Verification items for the finished model (mm, model axes). Face numbers are marked on the shaded views. A direction names the side the tool comes from. Give positions to 0.01 mm unless a question says otherwise; leave off trailing zeros. Write each loop counter-clockwise with the first axis right and the second up, starting at its lowest first coordinate (ties: lowest second). Pieces come first, ordered by that corner, then holes. Notation, with made-up numbers: (-14, -24) - (44, -24) arc R38 ccw to (44, 14) - close; hole circle Ø5 at (22.5, 31.5). An arc over 180 degrees is marked (long way). Answer as a JSON object with one key per item and string values. Group by question number.
Item 1: Sectioned sample at A-A, the plane x = -38. Record the boundary of the cut face in (y, z) (3 decimals), and give its area (3 significant figures).
Item 2: Draft check along Y on the marked faces 1, 2, 3 and 4. Enter one of: +Y half, -Y half, draft (parallel to the pull), parting line (faces both ways), or undercut.
Item 3: Scan lines: line 1 along Y through (x, z) = (-58, 29.5) (3 decimals); line 2 along Y through (x, z) = (-23, -48) (3 decimals); line 3 along X through (y, z) = (48.5, -33.5). Record each from-to range of solid material in increasing order. Write a range as [from, to].
Item 4: Sectioned sample at C-C, the plane x = -65.5. Record the boundary of the cut face in (y, z).
Item 5: Go/stop test with flat-tipped pins: pin 1 (1 mm diameter, centred on y = 69.5, z = 2, fed in from +X); pin 2 (16.5 mm diameter, centred on x = -52.39, z = 51.59, fed in from +Y); pin 3 (1.6 mm diameter, centred on y = 68.5, z = -47, fed in from +X) (3 decimals); pin 4 (7.5 mm diameter, centred on x = -28.58, z = 54.77, fed in from -Y). Record where each tip stops, or that it passes through.
Item 6: Tool access check on the marked faces 5 and 6. Record the directions out of +Z, -Z, +X, -X, +Y, -Y that give a thin tool (end or side, any length) a straight path to the whole face; none if there is none.
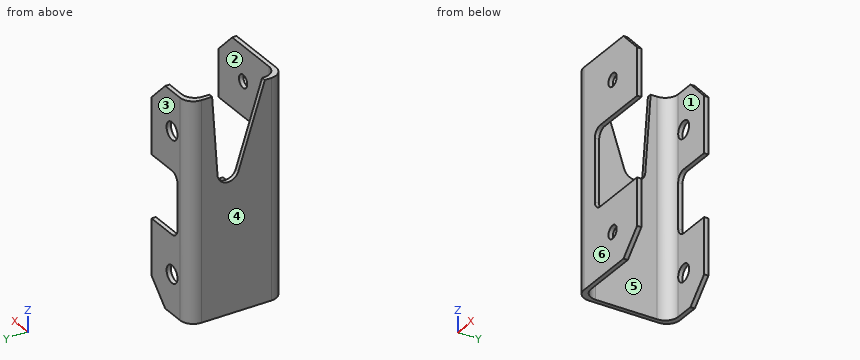
```python
from build123d import *

# Parameters (mm, degrees)
BOSS_EXTRUDE1_DEPTH = 80.16875
CUT_EXTRUDE2_DEPTH  = 4.175
CUT_EXTRUDE3_REACH  = 72.644
SKETCH3_R           = 6.35
CUT_EXTRUDE4_REACH  = 5.175
SKETCH4_R           = 4.7625


with BuildPart() as part:
    # Sketch1 → Boss-Extrude1 (new body, symmetric)
    with BuildSketch(Plane.XY):
        with BuildLine():
            Line((0, 0), (-61.9125, 0))
            ThreePointArc((-61.9125, 0), (-68.647692091, 2.789807909), (-71.4375, 9.525))
            Line((-71.4375, 9.525), (-71.4375, 61.11875))
            ThreePointArc((-71.4375, 61.11875), (-68.647692091, 67.853942091), (-61.9125, 70.64375))
            Line((-61.9125, 70.64375), (-28.575, 70.64375))
            Line((-28.575, 70.64375), (-28.575, 67.46875))
            Line((-28.575, 67.46875), (-58.7375, 67.46875))
            ThreePointArc((-58.7375, 67.46875), (-65.472692091, 64.678942091), (-68.2625, 57.94375))
            Line((-68.2625, 57.94375), (-68.2625, 12.7))
            ThreePointArc((-68.2625, 12.7), (-65.472692091, 5.964807909), (-58.7375, 3.175))
            Line((-58.7375, 3.175), (0, 3.175))
            Line((0, 3.175), (0, 0))
        make_face()
    extrude(amount=BOSS_EXTRUDE1_DEPTH, both=True)

    # Sketch2 → Cut-Extrude2 (cut, through all)
    with BuildSketch(Plane(origin=(-68.2625, 0, 0), x_dir=(0, 0, -1), z_dir=(1, 0, 0))):
        with BuildLine():
            Line((-22.471470052, 49.193610415), (-80.16875, 53.18125))
            Line((-80.16875, 53.18125), (-80.16875, 14.2875))
            Line((-80.16875, 14.2875), (-20.557643239, 33.728685684))
            ThreePointArc((-20.557643239, 33.728685684), (-15.141341042, 42.249850944), (-22.471470052, 49.193610415))
        make_face()
    extrude(amount=-CUT_EXTRUDE2_DEPTH, mode=Mode.SUBTRACT)

    # Sketch3 → Cut-Extrude3 (cut, up to next)
    with BuildSketch(Plane(origin=(0, 70.64375, 0), x_dir=(1, 0, 0), z_dir=(0, 1, 0)), mode=Mode.PRIVATE) as cut_extrude3_sk1:
        with Locations((-52.3875, 51.59375)):
            Circle(SKETCH3_R)
    cut_extrude3_tool1 = extrude(cut_extrude3_sk1.sketch, amount=-CUT_EXTRUDE3_REACH, mode=Mode.PRIVATE) & part.part
    add(cut_extrude3_tool1.solids().sort_by_distance((-52.3875, 70.64375, -51.59375))[0], mode=Mode.SUBTRACT)
    # Sketch3 → Cut-Extrude3 (cut, up to next)
    with BuildSketch(Plane(origin=(0, 70.64375, 0), x_dir=(1, 0, 0), z_dir=(0, 1, 0)), mode=Mode.PRIVATE) as cut_extrude3_sk2:
        with Locations((-52.3875, -51.59375)):
            Circle(SKETCH3_R)
    cut_extrude3_tool2 = extrude(cut_extrude3_sk2.sketch, amount=-CUT_EXTRUDE3_REACH, mode=Mode.PRIVATE) & part.part
    add(cut_extrude3_tool2.solids().sort_by_distance((-52.3875, 70.64375, 51.59375))[0], mode=Mode.SUBTRACT)
    # Sketch3 → Cut-Extrude3 (cut, up to next)
    with BuildSketch(Plane(origin=(0, 70.64375, 0), x_dir=(1, 0, 0), z_dir=(0, 1, 0)), mode=Mode.PRIVATE) as cut_extrude3_sk3:
        Polygon((-44.45, 80.16875), (-28.575, 64.29375), (-28.575, 80.16875), align=None)
    cut_extrude3_tool3 = extrude(cut_extrude3_sk3.sketch, amount=-CUT_EXTRUDE3_REACH, mode=Mode.PRIVATE) & part.part
    add(cut_extrude3_tool3.solids().sort_by_distance((-33.866667, 70.64375, -74.877083))[0], mode=Mode.SUBTRACT)
    # Sketch3 → Cut-Extrude3 (cut, up to next)
    with BuildSketch(Plane(origin=(0, 70.64375, 0), x_dir=(1, 0, 0), z_dir=(0, 1, 0)), mode=Mode.PRIVATE) as cut_extrude3_sk4:
        Polygon((-28.575, -80.16875), (-28.575, -64.29375), (-44.45, -80.16875), align=None)
    cut_extrude3_tool4 = extrude(cut_extrude3_sk4.sketch, amount=-CUT_EXTRUDE3_REACH, mode=Mode.PRIVATE) & part.part
    add(cut_extrude3_tool4.solids().sort_by_distance((-33.866667, 70.64375, 74.877083))[0], mode=Mode.SUBTRACT)
    # Sketch3 → Cut-Extrude3 (cut, up to next)
    with BuildSketch(Plane(origin=(0, 70.64375, 0), x_dir=(1, 0, 0), z_dir=(0, 1, 0)), mode=Mode.PRIVATE) as cut_extrude3_sk5:
        Polygon((-15.875, 80.16875), (0, 64.29375), (0, 80.16875), align=None)
    cut_extrude3_tool5 = extrude(cut_extrude3_sk5.sketch, amount=-CUT_EXTRUDE3_REACH, mode=Mode.PRIVATE) & part.part
    add(cut_extrude3_tool5.solids().sort_by_distance((-5.291667, 70.64375, -74.877083))[0], mode=Mode.SUBTRACT)
    # Sketch3 → Cut-Extrude3 (cut, up to next)
    with BuildSketch(Plane(origin=(0, 70.64375, 0), x_dir=(1, 0, 0), z_dir=(0, 1, 0)), mode=Mode.PRIVATE) as cut_extrude3_sk6:
        Polygon((-15.875, -80.16875), (0, -80.16875), (0, -64.29375), align=None)
    cut_extrude3_tool6 = extrude(cut_extrude3_sk6.sketch, amount=-CUT_EXTRUDE3_REACH, mode=Mode.PRIVATE) & part.part
    add(cut_extrude3_tool6.solids().sort_by_distance((-5.291667, 70.64375, 74.877083))[0], mode=Mode.SUBTRACT)
    # Sketch3 → Cut-Extrude3 (cut, up to next)
    with BuildSketch(Plane(origin=(0, 70.64375, 0), x_dir=(1, 0, 0), z_dir=(0, 1, 0)), mode=Mode.PRIVATE) as cut_extrude3_sk7:
        with BuildLine():
            Line((-28.575, 23.01875), (-28.575, -23.01875))
            Line((-28.575, -23.01875), (-52.3875, -23.01875))
            ThreePointArc((-52.3875, -23.01875), (-56.877628061, -21.158878061), (-58.7375, -16.66875))
            Line((-58.7375, -16.66875), (-58.7375, 16.66875))
            ThreePointArc((-58.7375, 16.66875), (-56.877628061, 21.158878061), (-52.3875, 23.01875))
            Line((-52.3875, 23.01875), (-28.575, 23.01875))
        make_face()
    cut_extrude3_tool7 = extrude(cut_extrude3_sk7.sketch, amount=-CUT_EXTRUDE3_REACH, mode=Mode.PRIVATE) & part.part
    add(cut_extrude3_tool7.solids().sort_by_distance((-43.483817, 70.64375, 0))[0], mode=Mode.SUBTRACT)

    # Sketch4 → Cut-Extrude4 (cut, up to next)
    with BuildSketch(Plane(origin=(0, 3.175, 0), x_dir=(1, 0, 0), z_dir=(0, 1, 0)), mode=Mode.PRIVATE) as cut_extrude4_sk1:
        with Locations((-28.575, 54.76875)):
            Circle(SKETCH4_R)
    cut_extrude4_tool1 = extrude(cut_extrude4_sk1.sketch, amount=-CUT_EXTRUDE4_REACH, mode=Mode.PRIVATE) & part.part
    add(cut_extrude4_tool1.solids().sort_by_distance((-28.575, 3.175, -54.76875))[0], mode=Mode.SUBTRACT)
    # Sketch4 → Cut-Extrude4 (cut, up to next)
    with BuildSketch(Plane(origin=(0, 3.175, 0), x_dir=(1, 0, 0), z_dir=(0, 1, 0)), mode=Mode.PRIVATE) as cut_extrude4_sk2:
        with Locations((-28.575, -54.76875)):
            Circle(SKETCH4_R)
    cut_extrude4_tool2 = extrude(cut_extrude4_sk2.sketch, amount=-CUT_EXTRUDE4_REACH, mode=Mode.PRIVATE) & part.part
    add(cut_extrude4_tool2.solids().sort_by_distance((-28.575, 3.175, 54.76875))[0], mode=Mode.SUBTRACT)
    # Sketch4 → Cut-Extrude4 (cut, up to next)
    with BuildSketch(Plane(origin=(0, 3.175, 0), x_dir=(1, 0, 0), z_dir=(0, 1, 0)), mode=Mode.PRIVATE) as cut_extrude4_sk3:
        with BuildLine():
            Line((0, 29.36875), (-42.8625, 29.36875))
            ThreePointArc((-42.8625, 29.36875), (-47.352628061, 27.508878061), (-49.2125, 23.01875))
            Line((-49.2125, 23.01875), (-49.2125, -23.01875))
            ThreePointArc((-49.2125, -23.01875), (-47.352628061, -27.508878061), (-42.8625, -29.36875))
            Line((-42.8625, -29.36875), (0, -29.36875))
            Line((0, -29.36875), (0, 29.36875))
        make_face()
    cut_extrude4_tool3 = extrude(cut_extrude4_sk3.sketch, amount=-CUT_EXTRUDE4_REACH, mode=Mode.PRIVATE) & part.part
    add(cut_extrude4_tool3.solids().sort_by_distance((-24.466585, 3.175, 0))[0], mode=Mode.SUBTRACT)


solid = part.part
```
Geometry check:
{
 "1": {"outline": "(0, -80.169) - (3.175, -80.169) - (3.175, -29.369) - (0, -29.369) - close; (0, 29.369) - (3.175, 29.369) - (3.175, 80.169) - (0, 80.169) - close; (67.469, -73.719) - (70.644, -73.719) - (70.644, -23.019) - (67.469, -23.019) - close; (67.469, 23.019) - (70.644, 23.019) - (70.644, 73.719) - (67.469, 73.719) - close", "area": "645 mm^2"},
 "2": {"face 1": "undercut", "face 2": "undercut", "face 3": "+Y half", "face 4": "draft"},
 "3": {"line 1": "[0, 3.175], [67.469, 70.644]", "line 2": "[0, 3.175]", "line 3": "[-71.44, -68.26]"},
 "4": {"outline": "(0.7, -80.17) - (5.99, -80.17) - (5.99, 80.17) - (0.7, 80.17) - close; (64.65, -80.17) - (69.94, -80.17) - (69.94, 80.17) - (64.65, 80.17) - close"},
 "5": {"pin 1": "x = -58.74", "pin 2": "y = 70.64", "pin 3": "x = -28.575", "pin 4": "y = 67.47"},
 "6": {"face 5": "+Z, -Z, +X", "face 6": "+Z, -Z, +X, -X, -Y"}
}
